Job drawing, mm, ordinate dimensions from the low corner. One solid piece. A direction names the side the tool comes from. Coordinates: 2 decimals unless noted, no trailing zeros. Loops run counter-clockwise (first coordinate to the right, second up) from the corner with the lowest first, then second, coordinate; pieces in that order, holes last. Notation, with made-up numbers: M -20.75,10 L 15.25,10 A19 ccw 15.25,20 Z; hole C 41.5,-10.75 d1. An arc over 180 degrees is marked long. Answer as a JSON object with one key per item and string values. Group by question number.
1. Saw through at D-D on x = 30. Write the cut outline in (y, z).
2. Saw through at C-C on y = 3. Write the cut outline in (x, z).
3. Mould opens along X. For the marked faces 1, 2 and 3 say: released by +X, released by -X, zero draft, split by the parting line, or undercut.
4. Saw through at B-B on z = 10. Write the cut outline in (x, y).
5. Drill centre lines: L1, parallel to X at y = 1.15, z = 10; L2, parallel to Z at x = 10, y = 6.35; L3, parallel to X at y = 4.75, z = 8.75. Where is each one in solid material? Low to high.
6. 3-axis set-ups, long thin cutter, end or side, ignore diameter. For the marked faces 4, 5 and 6: which of +Z, -Z, +X, -X, +Y, -Y reach the whole face in a straight line?
7. Saw through at A-A on x = 10. Write the cut outline in (y, z), then the cut area to 3 significant figures.
8. Drop flat-ended pins along their axis: pin 1 Ø12 at (x, z) = (10, 10) entering from -Y; pin 2 Ø5 at (x, z) = (29.5, 12) entering from +Y; pin 3 Ø1.5 at (y, z) = (5, 2.5) entering from +X. Give the stop position or say it passes through.
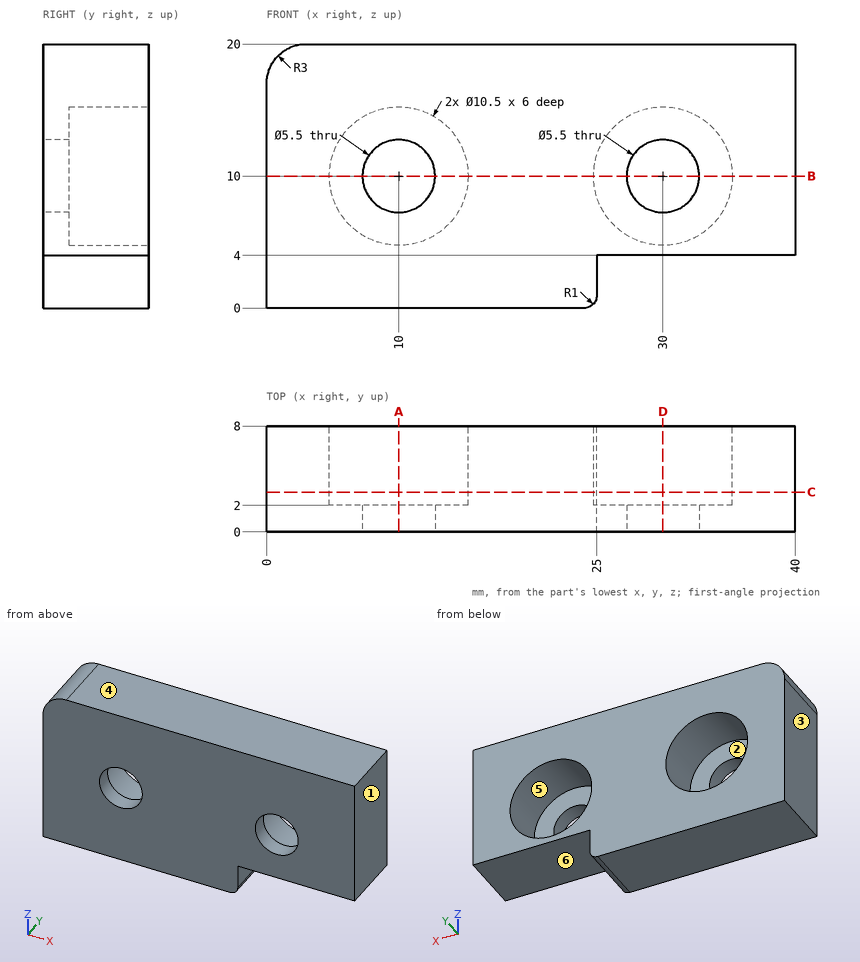
Outcome:
{
 "1": {"outline": "M 0,4 L 8,4 L 8,4.75 L 2,4.75 L 2,7.25 L 0,7.25 Z; M 0,12.75 L 2,12.75 L 2,15.25 L 8,15.25 L 8,20 L 0,20 Z"},
 "2": {"outline": "M 0,0 L 24,0 A1 ccw 25,1 L 25,4 L 40,4 L 40,20 L 3,20 A3 ccw 0,17 Z; hole C 10,10 d10.5; hole C 30,10 d10.5"},
 "3": {"face 1": "released by +X", "face 2": "undercut", "face 3": "released by -X"},
 "4": {"outline": "M 0,0 L 7.25,0 L 7.25,2 L 4.75,2 L 4.75,8 L 0,8 Z; M 12.75,0 L 27.25,0 L 27.25,2 L 24.75,2 L 24.75,8 L 15.25,8 L 15.25,2 L 12.75,2 Z; M 32.75,0 L 40,0 L 40,8 L 35.25,8 L 35.25,2 L 32.75,2 Z"},
 "5": {"L1": "x = 0 to 7.25, 12.75 to 27.25, 32.75 to 40", "L2": "z = 0 to 4.75, 15.25 to 20", "L3": "x = 0 to 4.9, 15.1 to 24.9, 35.1 to 40"},
 "6": {"face 4": "+Z, +X, -X, +Y, -Y", "face 5": "+Y", "face 6": "-Z, +X, +Y, -Y"},
 "7": {"outline": "M 0,0 L 8,0 L 8,4.75 L 2,4.75 L 2,7.25 L 0,7.25 Z; M 0,12.75 L 2,12.75 L 2,15.25 L 8,15.25 L 8,20 L 0,20 Z", "area": "86.0 mm²"},
 "8": {"pin 1": "stops at y = 0", "pin 2": "stops at y = 2", "pin 3": "stops at x = 25"}
}
